Verification items for the finished model (mm, model axes). A direction names the side the tool comes from. Round coordinates to 2 decimals unless told otherwise and drop trailing zeros. Write each loop counter-clockwise with the first axis right and the second up, starting at its lowest first coordinate (ties: lowest second). Pieces come first, ordered by that corner, then holes. Notation, with made-up numbers: (-1.5, 60.5) - (5.5, 60.5) arc R20 cw to (5.5, 94.5) - close; hole circle Ø8 at (42, 85). An arc over 180 degrees is marked (long way). Answer as a JSON object with one key per item and string values.
```python
from build123d import *

# Parameters (mm, degrees)
F0_W      = 348.996
F0_H      = 247.65
F0_R      = 3.81
F0_W_2    = 300.228
F0_H_2    = 200.406
F1_DEPTH  = 2.54
F2_W      = 304.292
F2_H      = 204.47
F2_W_2    = 300.228
F2_H_2    = 200.406
F3_DEPTH  = 101.6
F5_DEPTH  = 25.4
F6_W      = 19.05
F6_H      = 8.89
F7_DEPTH  = 8.89
F8_DEPTH  = 2.54
F10_D     = 9.525
F10_DEPTH = 12.7
F10_TIP   = 2.8615986981


with BuildPart() as f1:
    # F0 (on Top) → F1 (new body)
    with BuildSketch(Plane.XY):
        Rectangle(F0_W, F0_H)
        with Locations((-163.83, -112.014)):
            Circle(F0_R, mode=Mode.SUBTRACT)
        with Locations((-54.102, -112.014)):
            Circle(F0_R, mode=Mode.SUBTRACT)
        with Locations((-163.83, -1.27)):
            Circle(F0_R, mode=Mode.SUBTRACT)
        with Locations((54.356, -112.014)):
            Circle(F0_R, mode=Mode.SUBTRACT)
        with Locations((162.56, -112.014)):
            Circle(F0_R, mode=Mode.SUBTRACT)
        with Locations((162.56, -1.27)):
            Circle(F0_R, mode=Mode.SUBTRACT)
        with Locations((-163.83, 109.474)):
            Circle(F0_R, mode=Mode.SUBTRACT)
        with Locations((-54.102, 109.474)):
            Circle(F0_R, mode=Mode.SUBTRACT)
        Rectangle(F0_W_2, F0_H_2, mode=Mode.SUBTRACT)
        with Locations((54.356, 109.474)):
            Circle(F0_R, mode=Mode.SUBTRACT)
        with Locations((162.56, 109.474)):
            Circle(F0_R, mode=Mode.SUBTRACT)
    extrude(amount=F1_DEPTH)

    # F2 (on face) → F3 (join)
    with BuildSketch(Plane.XY.offset(2.54)):
        Rectangle(F2_W, F2_H)
        Rectangle(F2_W_2, F2_H_2, mode=Mode.SUBTRACT)
    extrude(amount=F3_DEPTH)

    # F4 (on face) → F5 (cut)
    with BuildSketch(Plane.XZ.offset(102.235)):
        with BuildLine():
            Line((122.936, 95.25), (122.936, 85.09))
            ThreePointArc((122.936, 85.09), (126.746, 81.28), (130.556, 85.09))
            Line((130.556, 85.09), (130.556, 95.25))
            ThreePointArc((130.556, 95.25), (126.746, 99.06), (122.936, 95.25))
        make_face()
        with BuildLine():
            Line((-130.556, 95.25), (-130.556, 85.09))
            ThreePointArc((-130.556, 85.09), (-126.746, 81.28), (-122.936, 85.09))
            Line((-122.936, 85.09), (-122.936, 95.25))
            ThreePointArc((-122.936, 95.25), (-126.746, 99.06), (-130.556, 95.25))
        make_face()
    extrude(amount=-F5_DEPTH, mode=Mode.SUBTRACT)

    # F6 (on face) → F7 (join)
    with BuildSketch(Plane.XZ.offset(-100.203)):
        with Locations((-89.789, 67.945)):
            Rectangle(F6_W, F6_H)
        with Locations((89.789, 67.945)):
            Rectangle(F6_W, F6_H)
    extrude(amount=F7_DEPTH)

    # F8 (add): a face of the model
    f8_faces = [f1.faces().sort_by_distance(p)[0] for p in [
        (0, -123.825, 1.27),
    ]]
    extrude(f8_faces, amount=F8_DEPTH)

    # F10
    with Locations(Plane(origin=(0, 102.235, 0), x_dir=(-1, 0, 0), z_dir=(0, 1, 0))):
        with Locations((0, 85.09)):
            Hole(F10_D / 2, depth=F10_DEPTH)
            with Locations((0, 0, -(F10_DEPTH + F10_TIP / 2))):  # 118° drill point
                Cone(0, F10_D / 2, F10_TIP, mode=Mode.SUBTRACT)


solid = f1.part
```
1. Material ranges on probe 1 along X at (y, z) = (-76.5, 18.5); probe 2 along Y at (x, z) = (-59, 47.5) (3 decimals); probe 3 along Y at (x, z) = (162.56, 0.9) (3 decimals), recorded low to high. Write a range as from..to.
Completed:
{"probe 1": "x = -152.15..-150.11, 150.11..152.15", "probe 2": "y = -102.235..-100.203, 100.203..102.235", "probe 3": "y = -126.365..-115.824, -108.204..-5.08, 2.54..105.664, 113.284..123.825"}
2. Go/stop test with flat-tipped pins: pin 1 (0.6 mm diameter, centred on y = -101.5, z = 91.5, fed in from +X); pin 2 (12 mm diameter, centred on x = -25, z = 82, fed in from +Y) (3 decimals); pin 3 (2.5 mm diameter, centred on x = 85.5, z = 68, fed in from -Y) (3 decimals). Record where each tip stops, or that it passes through.
Completed:
{"pin 1": "stops at x = 152.15", "pin 2": "stops at y = 102.235", "pin 3": "stops at y = -102.235"}
3. Access from +Z, -Z, +X, -X, +Y, -Y to the whole of each face (thin tool, end or side, straight path). Record for faces 4 (the face through (90, 96, 72.39)), 5 (the face through (-0.62, 101.2, 89.81)), 6 (the face through (99.314, 96, 68)).
Completed:
{"face 4": "+Z", "face 5": "+Y", "face 6": "+Z, -Z"}
4. Cross-section at A-A (x = 0). Record the boundary of the cut face in (y, z) (1 decimal).
Completed:
{"outline": "(-126.4, 0) - (-100.2, 0) - (-100.2, 104.1) - (-102.2, 104.1) - (-102.2, 2.5) - (-126.4, 2.5) - close; (100.2, 0) - (123.8, 0) - (123.8, 2.5) - (102.2, 2.5) - (102.2, 80.3) - (100.2, 80.3) - close; (100.2, 89.9) - (102.2, 89.9) - (102.2, 104.1) - (100.2, 104.1) - close"}
5. Cross-section at C-C (x = -43.5). Record the boundary of the cut face in (y, z) (3 decimals).
Completed:
{"outline": "(-126.365, 0) - (-100.203, 0) - (-100.203, 104.14) - (-102.235, 104.14) - (-102.235, 2.54) - (-126.365, 2.54) - close; (100.203, 0) - (123.825, 0) - (123.825, 2.54) - (102.235, 2.54) - (102.235, 104.14) - (100.203, 104.14) - close"}
6. Cross-section at D-D (z = 7). Record the boundary of the cut face in (x, y) (3 decimals).
Completed:
{"outline": "(-152.146, -102.235) - (152.146, -102.235) - (152.146, 102.235) - (-152.146, 102.235) - close; hole (-150.114, -100.203) - (150.114, -100.203) - (150.114, 100.203) - (-150.114, 100.203) - close"}
7. Cross-section at B-B (y = 83). Record the boundary of the cut face in (x, z).
Completed:
{"outline": "(-174.5, 0) - (-150.11, 0) - (-150.11, 104.14) - (-152.15, 104.14) - (-152.15, 2.54) - (-174.5, 2.54) - close; (150.11, 0) - (174.5, 0) - (174.5, 2.54) - (152.15, 2.54) - (152.15, 104.14) - (150.11, 104.14) - close"}
8. Mould release check, pull along Y, two halves, no side actions. Record for faces 1 (the face through (159.752, 112.049, 1.252)), 2 (the face through (-2, 102.235, 53)), 3 (the face through (-2, -102.235, 53)): released by +Y, released by -Y, zero draft, split by the parting line, or undercut.
Completed:
{"face 1": "undercut", "face 2": "released by +Y", "face 3": "released by -Y"}
